Geometry: final body of the model. Coordinates: model frame, mm. A direction names the side the tool comes from. Coordinates: 2 decimals unless noted, no trailing zeros. Order: outer loops, then holes, each group sorted by start corner. A loop starts at its lowest first (then second) coordinate and runs counter-clockwise, first axis right, second up. Notation, with made-up numbers: M 13.5,76.5 L 46.5,76.5 A19 ccw 46.5,110.5 Z; hole C -19.5,26 d3. An arc over 180 degrees is marked long. Use CSV: the item, a comma, the result in double quotes. Start each with the question number.
1. First-contact query: P1, Ø6, axis at y = 8, z = -12, coming from the -X side; P2, Ø3, axis at y = 10, z = -16.5, coming from the +X side; P3, Ø5, axis at x = 8.5, y = 11.5, coming from the -Z side. Flat tips, straight axial feed; report the tip coordinate or a pass-through.
2. Section query A-A on y = 12.25. Return the cut outline in (x, z), and give its area (3 significant figures).
3. Section query C-C on x = 3.5. Return the cut outline in (y, z), and give its area (3 significant figures).
4. Material intervals for line 1 (Y direction, x = 12, z = 0.9); line 2 (X direction, y = 7, z = -18); line 3 (Z direction, x = 11.5, y = 2), sorted ascending.
5. Pull-direction query (X, two-part tool) for faces 3 (the flat face through (2.8, 16, 0.2)), 4 (the cylindrical face through (11.46, 5.56, 1.01)), 5 (the cylindrical face through (-0.93, 8.11, 0.9)); classes: pulls with the +X half, pulls with the -X half, needs draft (parallel to the pull), parting line crosses it, or undercut.
6. Set-up query: faces 1 (the flat face through (0, 8, -8)), 2 (the flat face through (2.8, 0, 0.2)). Return all of +Z, -Z, +X, -X, +Y, -Y with unobstructed straight access to the full face (end or side cutting, diameter ignored); none if empty.
7. Section query B-B on z = -2. Return the cut outline in (x, y).
from build123d import *

# Parameters (mm, degrees)
EXTRUDE_1_DEPTH     = 16
FILLET_1_R          = 8
SKETCH_2_R          = 2.5
CUT_EXTRUDE_1_DEPTH = 16
SKETCH_3_R          = 2.5
CUT_EXTRUDE_2_DEPTH = 16
FILLET_3_R          = 2
FILLET_4_R          = 0.5
CHAMFER_1_SIZE      = 0.5


with BuildPart() as part:
    # Эскиз1 → Бобышка-Вытянуть1 (new body)
    with BuildSketch(Plane(origin=(0, 0, 0), x_dir=(1, 0, 0), z_dir=(0, 1, 0))):
        Polygon((0, 20), (0, 0), (20, 0), (20, -1.5), (-1.5, -1.5), (-1.5, 20), align=None)
    extrude(amount=EXTRUDE_1_DEPTH)

    # Скругление1
    fillet_1_edges = [part.edges().sort_by_distance(p)[0] for p in [
        (-0.75, 0, -20),
        (-0.75, 16, -20),
        (20, 0, 0.75),
        (20, 16, 0.75),
    ]]
    fillet(fillet_1_edges, radius=FILLET_1_R - 0.0001)  # a hair under: the kernel refuses the full size

    # Эскиз2 → Вырез-Вытянуть1 (cut)
    with BuildSketch(Plane.XY.offset(1.5)):
        with Locations((12, 8)):
            Circle(SKETCH_2_R)
    extrude(amount=-CUT_EXTRUDE_1_DEPTH, mode=Mode.SUBTRACT)

    # Эскиз3 → Вырез-Вытянуть2 (cut)
    with BuildSketch(Plane.ZY.offset(1.5)):
        with Locations((-12, 8)):
            Circle(SKETCH_3_R)
    extrude(amount=-CUT_EXTRUDE_2_DEPTH, mode=Mode.SUBTRACT)

    # Скругление3
    fillet_3_edges = [part.edges().sort_by_distance(p)[0] for p in [
        (-1.5, 8, 1.5),
    ]]
    fillet(fillet_3_edges, radius=FILLET_3_R)

    # Скругление4
    fillet_4_edges = [part.edges().sort_by_distance(p)[0] for p in [
        (0, 8, 0),
    ]]
    fillet(fillet_4_edges, radius=FILLET_4_R)

    # Фаска1
    chamfer_1_edges = [part.edges().sort_by_distance(p)[0] for p in [
        (9.5, 8, 0),
        (0, 8, -14.5),
    ]]
    chamfer(chamfer_1_edges, length=CHAMFER_1_SIZE)


solid = part.part
Results list:
1,P1,"stops at x = -1.5"
1,P2,"stops at x = 0"
1,P3,"stops at z = 0"
2,outline,"M -1.5,-18.78 L 0,-18.78 L 0,-0.5 A0.5 cw 0.5,0 L 18.78,0 L 18.78,1.5 L 0.5,1.5 A2 ccw -1.5,-0.5 Z"
2,area,"57.8 mm²"
3,outline,"M 0,0 L 16,0 L 16,1.5 L 0,1.5 Z"
3,area,"24.0 mm²"
4,line 1,"y = 0 to 5.5, 10.5 to 16"
4,line 2,"x = -1.5 to 0"
4,line 3,"z = 0 to 1.5"
5,face 3,"needs draft"
5,face 4,"undercut"
5,face 5,"pulls with the -X half"
6,face 1,"-Z, +X, +Y, -Y"
6,face 2,"+Z, -Z, +X, -X, -Y"
7,outline,"M -1.5,0 L 0,0 L 0,16 L -1.5,16 Z"
